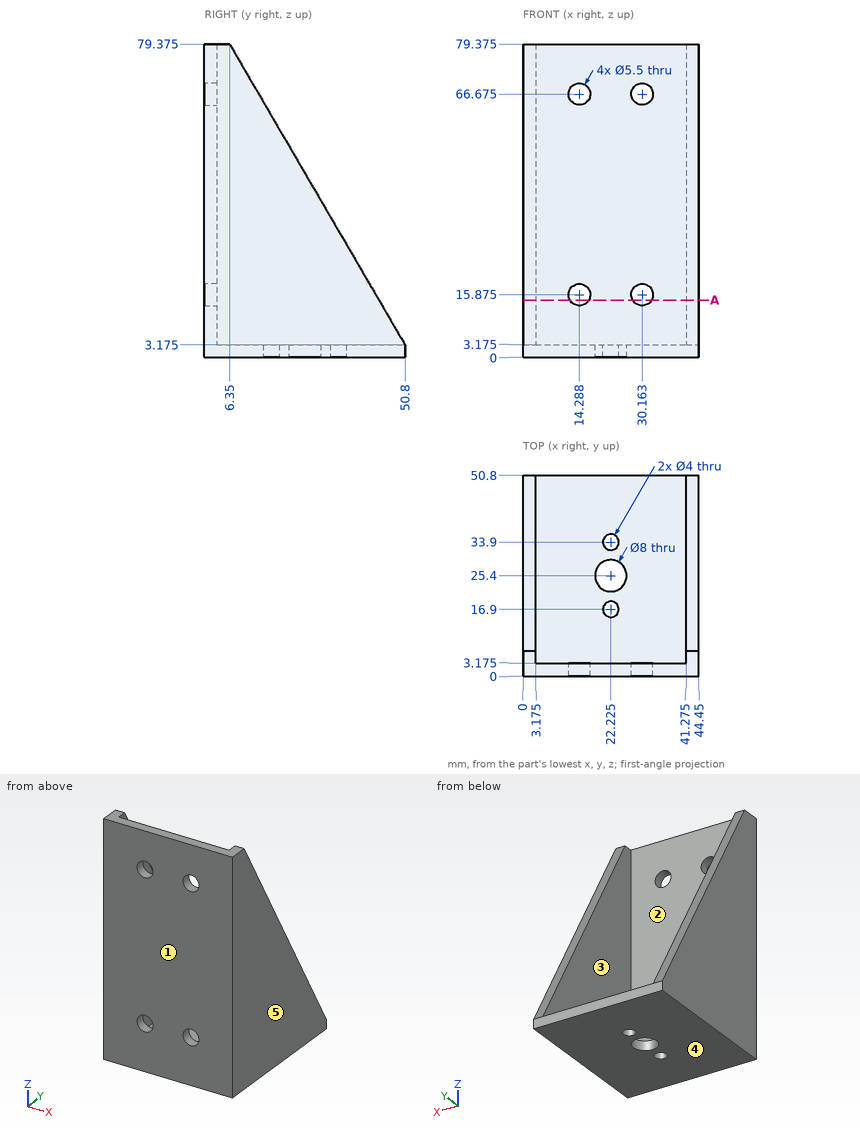
Geometry: see drawing. Coordinates: mm, zero at the bounding-box minimum. A direction names the side the tool comes from. Coordinates: 2 decimals unless noted, no trailing zeros. Use a Markdown table: item, result.
1) Pull-direction query (X, two-part tool) for the marked faces 3, 4 and 5; classes: released by +X, released by -X, zero draft, split by the parting line, or undercut.
Results found:
| item | result |
|---|---|
| face 3 | undercut |
| face 4 | zero draft |
| face 5 | released by +X |
2) Cut plane A-A (z = 14.5). Give the number of separate pieces and of enclosed holes in the cut face.
Results found:
| item | result |
|---|---|
| separate pieces | 3 |
| enclosed holes | 0 |
3) Material intervals for line 1 along Z through (x, y) = (21, 19) (1 decimal); line 2 along X through (y, z) = (33, 2), sorted ascending. Write a range as from..to.
Results found:
| item | result |
|---|---|
| line 1 | z = 0..3.2 |
| line 2 | x = 0..20.44, 24.01..44.45 |
4) Access query for the marked faces 1 and 2. Directions: +Z, -Z, +X, -X, +Y, -Y. A direction counts if a zero-diameter tool reaches every point of the face in a straight line with its end or side. Return the directions, or none.
Results found:
| item | result |
|---|---|
| face 1 | +Z, -Z, +X, -X, -Y |
| face 2 | +Z, +Y |
5) Contact query for flat-ended pins moving along their axis: pin 1 (3.5 mm diameter, centred on x = 14.29, z = 66.68, fed in from +Y); pin 2 (4 mm diameter, centred on x = 27.5, z = 11.5, fed in from +Y) (1 decimal); pin 3 (2 mm diameter, centred on x = 36, y = 30, fed in from +Z) (1 decimal). Output: stop coordinate, or through.
Results found:
| item | result |
|---|---|
| pin 1 | passes through |
| pin 2 | stops at y = 3.2 |
| pin 3 | stops at z = 3.2 |
